Answer from the drawing. Dimensions are ordinates in mm from the lowest x, y and z of the part. Coordinates: 2 decimals unless noted, no trailing zeros. Write each loop counter-clockwise with the first axis right and the second up, starting at its lowest first coordinate (ties: lowest second). Pieces come first, ordered by that corner, then holes.
(1) The part is cut by section C-C, the plane y = 53. Determine the outline of the cut face in (x, z), and give its area (3 significant figures).
(2) Straight lines are drawn through the part: line 1 along X through (y, z) = (29.5, 1.55); line 2 along Y through (x, z) = (37, 2.05); line 3 along Y through (x, z) = (22, 1.95). For each, find the intervals that lie inside material, in ascending order.
(3) The part is cut by section D-D, the plane x = 10. Determine the outline of the cut face in (y, z), and give its area (3 significant figures).
(4) Given pin 1 (1 mm diameter, centred on x = 6, z = 1.5, fed in from -Y); pin 2 (0.9 mm diameter, centred on y = 93.5, z = 1.5, fed in from -X); pin 3 (1.4 mm diameter, centred on x = 1, z = 1, fed in from +Y), each flat-ended and moving along its own axis, determine where each tip first touches the part or whether it passes through.
(5) The part is cut by section A-A, the plane x = 24. Determine the outline of the cut face in (y, z), and give its area (3 significant figures).
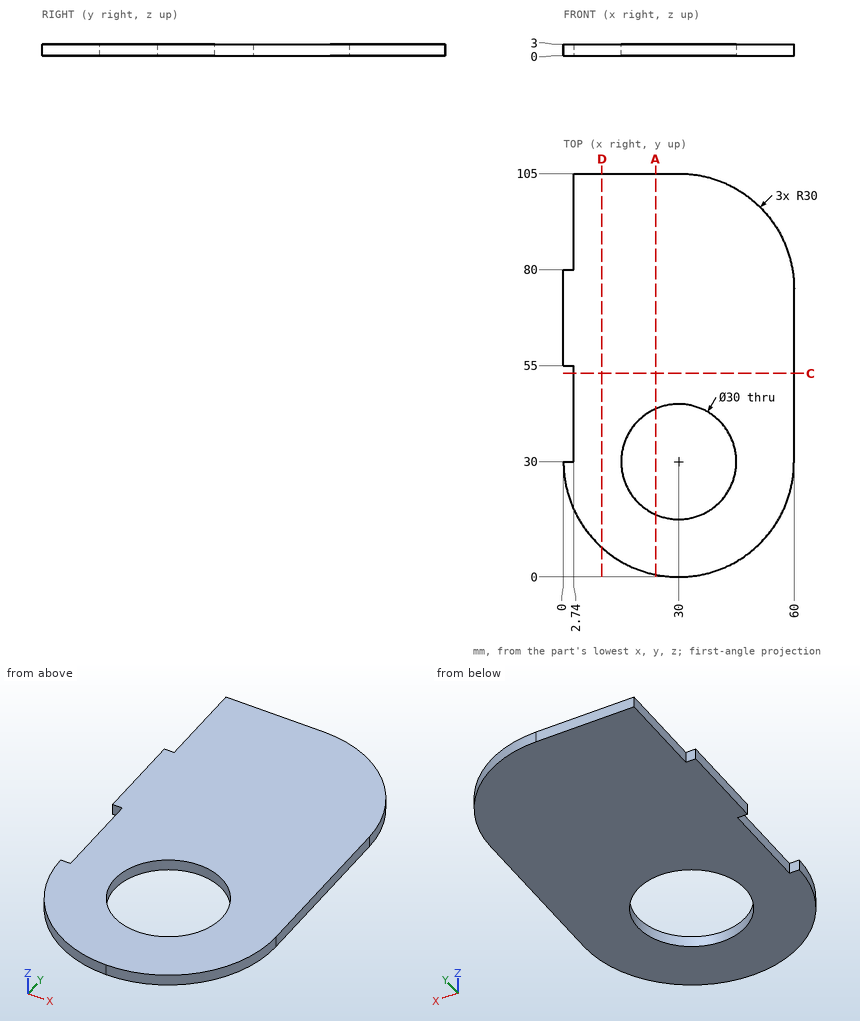
Computed:
1. outline: (2.74, 0) - (60, 0) - (60, 3) - (2.74, 3) - close
1. area: 172 mm2
2. line 1: x = 0 to 15.01, 44.99 to 60
2. line 2: y = 0.83 to 16.73, 43.27 to 104.17
2. line 3: y = 1.09 to 17.31, 42.69 to 105
3. outline: (7.64, 0) - (105, 0) - (105, 3) - (7.64, 3) - close
3. area: 292 mm2
4. pin 1: stops at y = 11.35
4. pin 2: stops at x = 2.74
4. pin 3: stops at y = 80
5. outline: (0.61, 0) - (16.25, 0) - (16.25, 3) - (0.61, 3) - close; (43.75, 0) - (105, 0) - (105, 3) - (43.75, 3) - close
5. area: 231 mm2
